Verification items for this drawing (mm, ordinates from the low corner). A direction names the side the tool comes from. Round coordinates to 2 decimals unless told otherwise and drop trailing zeros. Write each loop counter-clockwise with the first axis right and the second up, starting at its lowest first coordinate (ties: lowest second). Pieces come first, ordered by that corner, then holes. Notation, with made-up numbers: (65, 73) -> (122, 73) arc R12 cw to (122, 88) -> close; hole circle Ø3 at (-1, -20.75). An arc over 180 degrees is marked (long way). One line per question, with ' | ' between items.
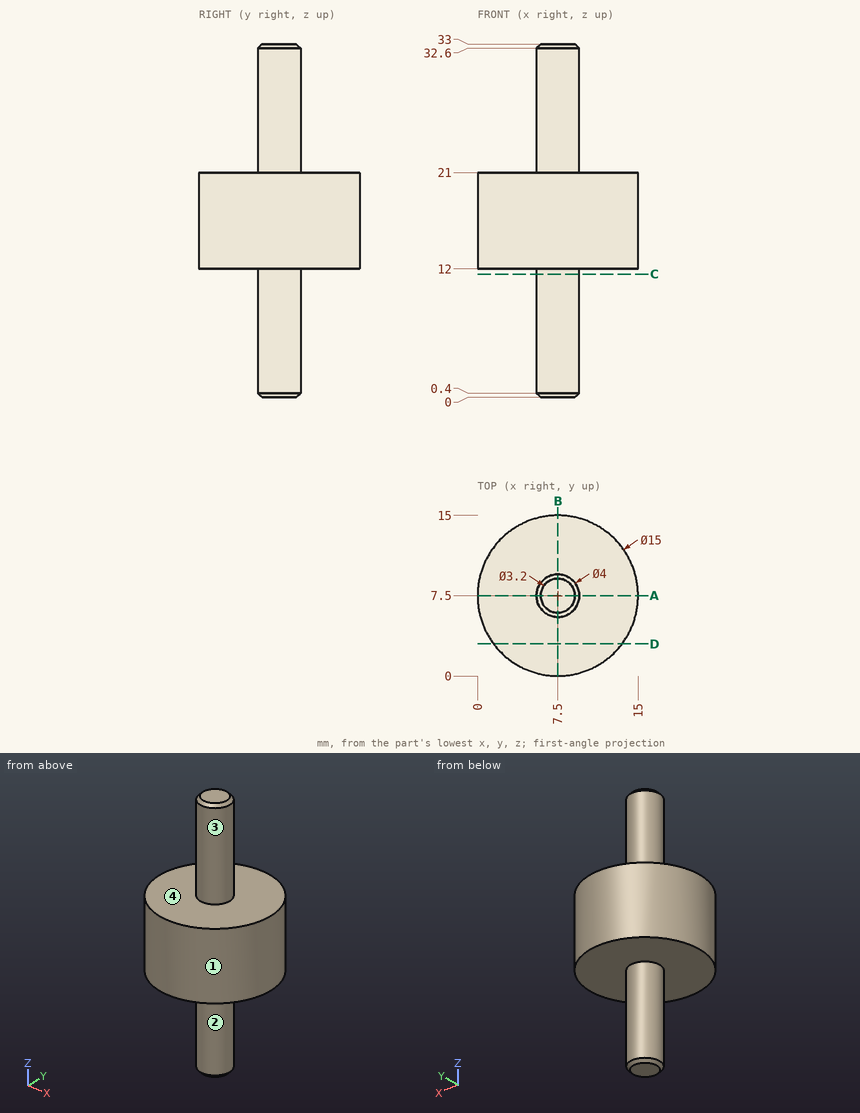
(1) Material ranges on line 1 (Z direction, x = 4, y = 7); line 2 (Y direction, x = 7.75, z = 20); line 3 (X direction, y = 1.25, z = 12.5), recorded low to high.
Resolved:
line 1: z = 12 to 21 | line 2: y = 0 to 15 | line 3: x = 3.35 to 11.65
(2) Sectioned sample at C-C on z = 11.5. Record the cut outline in (x, y).
Resolved:
outline: circle Ø4 at (7.5, 7.5)
(3) Draft check along X on the marked faces 3 and 4. Enter one of: +X half, -X half, draft (parallel to the pull), parting line (faces both ways), or undercut.
Resolved:
face 3: parting line | face 4: draft
(4) Sectioned sample at D-D on y = 3. Record the cut outline in (x, z), then the cut area to 3 significant figures.
Resolved:
outline: (1.5, 12) -> (13.5, 12) -> (13.5, 21) -> (1.5, 21) -> close | area: 108 mm2
(5) Go/stop test with flat-tipped pins: pin 1 (1.5 mm diameter, centred on x = 4.5, z = 25.5, fed in from +Y); pin 2 (5 mm diameter, centred on x = 8.5, y = 7, fed in from -Z); pin 3 (4 mm diameter, centred on y = 3.5, z = 11, fed in from -X); pin 4 (5 mm diameter, centred on x = 4, z = 25, fed in from +Y). Record where each tip stops, or that it passes through.
Resolved:
pin 1: passes through | pin 2: stops at z = 0 | pin 3: stops at x = 0.35 | pin 4: stops at y = 9.23
(6) Access from +Z, -Z, +X, -X, +Y, -Y to the whole of each face (thin tool, end or side, straight path). Record for the marked faces 1 and 2.
Resolved:
face 1: +Z, -Z | face 2: -Z
(7) Sectioned sample at A-A on y = 7.5. Record the cut outline in (x, z), then the cut area to 3 significant figures.
Resolved:
outline: (0, 12) -> (5.5, 12) -> (5.5, 0.4) -> (5.9, 0) -> (9.1, 0) -> (9.5, 0.4) -> (9.5, 12) -> (15, 12) -> (15, 21) -> (9.5, 21) -> (9.5, 32.6) -> (9.1, 33) -> (5.9, 33) -> (5.5, 32.6) -> (5.5, 21) -> (0, 21) -> close | area: 231 mm2
